Geometry: final body of the model. Coordinates: model frame, mm. Face numbers are marked on the shaded views. A direction names the side the tool comes from. Give positions to 0.01 mm unless a question says otherwise; leave off trailing zeros. Loops run counter-clockwise (first coordinate to the right, second up) from the corner with the lowest first, then second, coordinate; pieces in that order, holes last.
1. Section C-C, the plane z = -16.5. Output: boundary loops of the cut face in (x, y), then the cut area to 3 significant figures.
2. Draft query along Z for the marked faces 1, 2, 3 and 4. Return one class per face: +Z half, -Z half, draft (parallel to the pull), parting line (faces both ways), or undercut.
3. Material intervals for line 1 along X through (y, z) = (5.5, 55.75); line 2 along Z through (x, y) = (-11, 10); line 3 along X through (y, z) = (14.75, 24.5), sorted ascending.
4. Section A-A, the plane x = 1. Output: boundary loops of the cut face in (y, z).
5. Section D-D, the plane z = 38. Output: boundary loops of the cut face in (x, y), then the cut area to 3 significant figures.
6. Access query for the marked faces 5, 6 and 7. Directions: +Z, -Z, +X, -X, +Y, -Y. A direction counts if a zero-diameter tool reaches every point of the face in a straight line with its end or side. Return the directions, or none.
7. First-contact query: P1, Ø1.5, axis at x = 7.5, z = -30.5, coming from the +Y side; P2, Ø0.5, axis at x = 4.5, y = 20.5, coming from the -Z side; P3, Ø7.5, axis at x = -2, z = -10.5, coming from the -Y side. Flat tips, straight axial feed; report the tip coordinate or a pass-through.
8. Section B-B, the plane z = 55.75. Output: boundary loops of the cut face in (x, y), then the cut area to 3 significant figures.
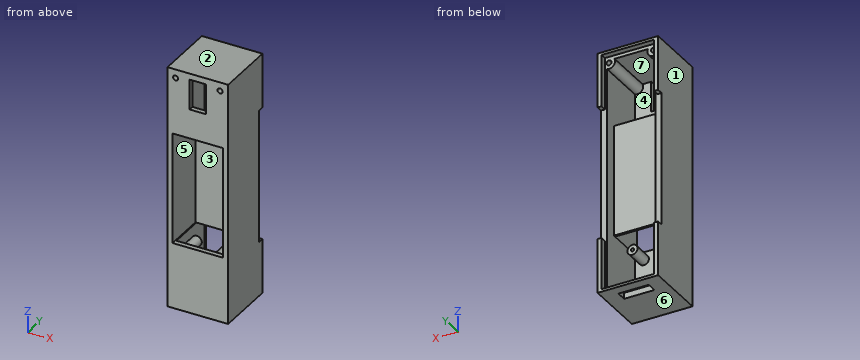
from build123d import *

# Parameters (mm, degrees)
SKETCH1_W                   = 30
SKETCH1_H                   = 120
BOSS_EXTRUDE1_DEPTH         = 30
SKETCH3_W                   = 24
SKETCH3_H                   = 114
CUT_EXTRUDE1_DEPTH          = 27.5
SKETCH4_W                   = 26
SKETCH4_H                   = 117.5
CUT_EXTRUDE2_DEPTH          = 3
SKETCH5_W                   = 66
SKETCH5_H                   = 3
CUT_EXTRUDE3_DEPTH          = 74.484692283
SKETCH6_W                   = 25
SKETCH6_H                   = 55
CUT_EXTRUDE4_DEPTH          = 20
SKETCH8_W                   = 24
SKETCH8_H                   = 55
BOSS_EXTRUDE2_DEPTH         = 1
SKETCH9_W                   = 15
SKETCH9_H                   = 5
CUT_EXTRUDE5_DEPTH          = 3
SKETCH10_R                  = 2.5
BOSS_EXTRUDE3_DEPTH         = 10
BOSS_EXTRUDE4_DEPTH         = 24.5
M2X0_4_TAPPED_HOLE1_D       = 1.6
M2X0_4_TAPPED_HOLE1_DEPTH   = 5.2
M2X0_4_TAPPED_HOLE1_TIP     = 0.480688495
TAP_DRILL_FOR_M3X0_5_TAP2_D = 2.5
SKETCH22_W                  = 8
SKETCH22_H                  = 15
CUT_EXTRUDE6_DEPTH          = 68.684931853


with BuildPart() as part:
    # Sketch1 → Boss-Extrude1 (new body)
    with BuildSketch(Plane(origin=(0, 0, 0), x_dir=(1, 0, 0), z_dir=(0, 1, 0))):
        Rectangle(SKETCH1_W, SKETCH1_H)
    extrude(amount=BOSS_EXTRUDE1_DEPTH)

    # Sketch3 → Cut-Extrude1 (cut)
    with BuildSketch(Plane(origin=(0, 30, 0), x_dir=(1, 0, 0), z_dir=(0, 1, 0))):
        Rectangle(SKETCH3_W, SKETCH3_H)
    extrude(amount=-CUT_EXTRUDE1_DEPTH, mode=Mode.SUBTRACT)

    # Sketch4 → Cut-Extrude2 (cut)
    with BuildSketch(Plane(origin=(0, 30, 0), x_dir=(1, 0, 0), z_dir=(0, 1, 0))):
        Rectangle(SKETCH4_W, SKETCH4_H)
    extrude(amount=-CUT_EXTRUDE2_DEPTH, mode=Mode.SUBTRACT)

    # Sketch5 → Cut-Extrude3 (cut, through all)
    with BuildSketch(Plane(origin=(15, 0, 0), x_dir=(0, 0, -1), z_dir=(1, 0, 0))):
        with Locations((0, 28.5)):
            Rectangle(SKETCH5_W, SKETCH5_H)
    extrude(amount=-CUT_EXTRUDE3_DEPTH, mode=Mode.SUBTRACT)

    # Sketch6 → Cut-Extrude4 (cut)
    with BuildSketch(Plane.XZ):
        Rectangle(SKETCH6_W, SKETCH6_H)
    extrude(amount=-CUT_EXTRUDE4_DEPTH, mode=Mode.SUBTRACT)

    # Sketch8 → Boss-Extrude2 (add)
    with BuildSketch(Plane.XZ.offset(-20)):
        Rectangle(SKETCH8_W, SKETCH8_H)
    extrude(amount=-BOSS_EXTRUDE2_DEPTH)

    # Sketch9 → Cut-Extrude5 (cut)
    with BuildSketch(Plane(origin=(0, 0, -60), x_dir=(-1, 0, 0), z_dir=(0, 0, -1))):
        with Locations((0, 22.5)):
            Rectangle(SKETCH9_W, SKETCH9_H)
    extrude(amount=-CUT_EXTRUDE5_DEPTH, mode=Mode.SUBTRACT)

    # Sketch10 → Boss-Extrude3 (add)
    with BuildSketch(Plane(origin=(0, 2.5, 0), x_dir=(1, 0, 0), z_dir=(0, 1, 0))):
        with Locations(Location((-7.62, 31.455, 0), (0, 0, 90))):
            Circle(SKETCH10_R)
        with Locations(Location((-7.62, 53.045, 0), (0, 0, 90))):
            Circle(SKETCH10_R)
        with Locations(Location((7.62, 53.045, 0), (0, 0, 90))):
            Circle(SKETCH10_R)
        with Locations(Location((7.62, 31.455, 0), (0, 0, 90))):
            Circle(SKETCH10_R)
    extrude(amount=BOSS_EXTRUDE3_DEPTH)

    # Sketch13 → Boss-Extrude4 (add)
    with BuildSketch(Plane(origin=(0, 27, 0), x_dir=(1, 0, 0), z_dir=(0, 1, 0))):
        with BuildLine():
            Line((-12, -52.921572875), (-12, -57))
            Line((-12, -57), (-8.272821971, -57))
            ThreePointArc((-8.272821971, -57), (-8.785462139, -53.726186258), (-12, -52.921572875))
        make_face()
        with BuildLine():
            Line((12, -57), (8.272821971, -57))
            ThreePointArc((8.272821971, -57), (8.785462139, -53.726186258), (12, -52.921572875))
            Line((12, -52.921572875), (12, -57))
        make_face()
    extrude(amount=-BOSS_EXTRUDE4_DEPTH)

    # M2x0.4 Tapped Hole1
    with Locations(Plane(origin=(0, 12.5, 0), x_dir=(1, 0, 0), z_dir=(0, 1, 0))):
        with Locations((-7.62, 31.455), (-7.62, 53.045), (7.62, 53.045), (7.62, 31.455)):
            Hole(M2X0_4_TAPPED_HOLE1_D / 2, depth=M2X0_4_TAPPED_HOLE1_DEPTH)
            with Locations((0, 0, -(M2X0_4_TAPPED_HOLE1_DEPTH + M2X0_4_TAPPED_HOLE1_TIP / 2))):  # 118° drill point
                Cone(0, M2X0_4_TAPPED_HOLE1_D / 2, M2X0_4_TAPPED_HOLE1_TIP, mode=Mode.SUBTRACT)

    # Tap Drill for M3x0.5 Tap2 (through all)
    with Locations(Plane(origin=(0, 27, 0), x_dir=(1, 0, 0), z_dir=(0, 1, 0))):
        with Locations((-11, -55.75), (11, -55.75)):
            Hole(TAP_DRILL_FOR_M3X0_5_TAP2_D / 2)

    # Sketch22 → Cut-Extrude6 (cut, through all)
    with BuildSketch(Plane(origin=(0, 2.5, 0), x_dir=(1, 0, 0), z_dir=(0, 1, 0))):
        with Locations((0, -49.5)):
            Rectangle(SKETCH22_W, SKETCH22_H)
    extrude(amount=-CUT_EXTRUDE6_DEPTH, mode=Mode.SUBTRACT)


solid = part.part
Answers below:
1. outline: (-15, 0) - (-12.5, 0) - (-12.5, 20) - (12.5, 20) - (12.5, 0) - (15, 0) - (15, 27) - (12, 27) - (12, 21) - (-12, 21) - (-12, 27) - (-15, 27) - close
1. area: 166 mm2
2. face 1: draft
2. face 2: +Z half
2. face 3: undercut
2. face 4: undercut
3. line 1: x = -15 to -12.25, -9.75 to -8, 8 to 9.75, 12.25 to 15
3. line 2: z = -60 to -57, 52.75 to 54.5, 57 to 60
3. line 3: x = -15 to -12.5, 12.5 to 15
4. outline: (0, -60) - (20, -60) - (20, -57) - (2.5, -57) - (2.5, -27.5) - (0, -27.5) - close; (0, 27.5) - (2.5, 27.5) - (2.5, 42) - (0, 42) - close; (0, 57) - (27, 57) - (27, 58.75) - (30, 58.75) - (30, 60) - (0, 60) - close; (20, -27.5) - (21, -27.5) - (21, 27.5) - (20, 27.5) - close; (25, -60) - (30, -60) - (30, -58.75) - (27, -58.75) - (27, -57) - (25, -57) - close
5. outline: (-15, 0) - (15, 0) - (15, 30) - (13, 30) - (13, 27) - (12, 27) - (12, 2.5) - (-12, 2.5) - (-12, 27) - (-13, 27) - (-13, 30) - (-15, 30) - close
5. area: 234 mm2
6. face 5: -Y
6. face 6: -Z, +X, -X, +Y, -Y
6. face 7: +Y
7. P1: stops at y = 12.5
7. P2: stops at z = -27.5
7. P3: stops at y = 20
8. outline: (-15, 0) - (-12.25, 0) - (-12.25, 27) - (-13, 27) - (-13, 30) - (-15, 30) - close; (-9.75, 0) - (-4, 0) - (-4, 2.5) - (-8, 2.5) - (-8, 27) - (-9.75, 27) - close; (4, 0) - (9.75, 0) - (9.75, 27) - (8, 27) - (8, 2.5) - (4, 2.5) - close; (12.25, 0) - (15, 0) - (15, 30) - (13, 30) - (13, 27) - (12.25, 27) - close
8. area: 275 mm2
